Geometry: see drawing. Coordinates: mm, zero at the bounding-box minimum. A direction names the side the tool comes from. Coordinates: 2 decimals unless noted, no trailing zeros. Write each loop counter-clockwise with the first axis right and the second up, starting at its lowest first coordinate (ties: lowest second). Pieces come first, ordered by that corner, then holes.
1) Section query C-C (x = 76). Output: boundary loops of the cut face in (y, z).
2) Section query A-A (z = 3). State how many separate pieces and enclosed holes the cut face has, then the cut area to 3 significant figures.
3) Section query B-B (y = 74.5). Output: boundary loops of the cut face in (x, z).
4) Pin query (flat end, axial travel): pin 1 Ø1.6 at (y, z) = (56, 5) entering from -X; pin 2 Ø5.5 at (x, y) = (42, 9.5) entering from +Z; pin 3 Ø1.5 at (y, z) = (49, 4.5) entering from -X; pin 4 Ø1.6 at (y, z) = (56, 7.5) entering from +X. Return the tip coordinate at first contact, or that it passes through.
5) Set-up query: the marked faces 1, 2 and 3. Return all of +Z, -Z, +X, -X, +Y, -Y with unobstructed straight access to the full face (end or side cutting, diameter ignored); none if empty.
6) Line query: L1, parallel to Y at x = 42, z = 2.25 (1 decimal); L2, parallel to Y at x = 41.5, z = 8.75 (1 decimal); L3, parallel to Z at x = 11, y = 28. Output: solid intervals per line, ascending.
7) Draft query along X for the marked faces 4, 5 and 6. Return one class per face: pulls with the +X half, pulls with the -X half, needs draft (parallel to the pull), parting line crosses it, or undercut.
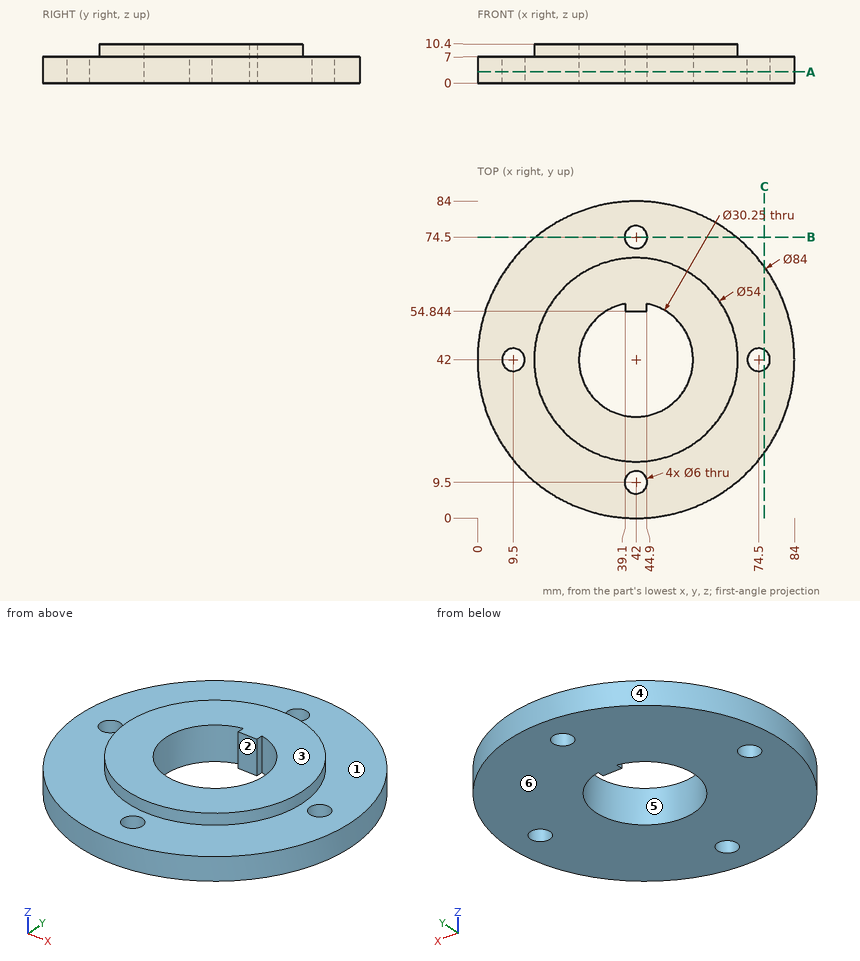
Answer:
1. outline: (17.34, 0) - (39.4, 0) - (39.4, 7) - (17.34, 7) - close; (44.6, 0) - (66.66, 0) - (66.66, 7) - (44.6, 7) - close
2. separate pieces: 1
2. enclosed holes: 5
2. area: 4,720 mm2
3. outline: (15.4, 0) - (39, 0) - (39, 7) - (15.4, 7) - close; (45, 0) - (68.6, 0) - (68.6, 7) - (45, 7) - close
4. pin 1: stops at x = 2.13
4. pin 2: passes through
4. pin 3: stops at x = 0.47
4. pin 4: stops at x = 81.81
5. face 1: +Z
5. face 2: +Z, -Z
5. face 3: +Z, +X, -X, +Y, -Y
6. L1: y = 0 to 6.5, 12.5 to 26.9, 54.8 to 71.5, 77.5 to 84
6. L2: y = 15 to 26.9, 54.8 to 69
6. L3: z = 0 to 7
7. face 4: parting line crosses it
7. face 5: undercut
7. face 6: needs draft
